```python
from build123d import *

# Parameters (mm, degrees)
F1_DEPTH = 10
F3_DEPTH = 10
F5_D     = 5
F5_DEPTH = 5
F5_TIP   = 1.5021515476


with BuildPart() as f1:
    # F0 (on Top) → F1 (new body)
    with BuildSketch(Plane.XY):
        with BuildLine():
            ThreePointArc((0, 17.5), (12.3743686708, 12.3743686708), (17.5, 0))
            ThreePointArc((17.5, 0), (12.3743686708, -12.3743686708), (0, -17.5))
            Line((0, -17.5), (0, -50))
            Line((0, -50), (150, -50))
            Line((150, -50), (150, 50))
            Line((150, 50), (0, 50))
            Line((0, 50), (0, 17.5))
        make_face()
        with BuildLine():
            ThreePointArc((0, -17.5), (-17.5, 0), (0, 17.5))
            Line((0, 17.5), (0, 50))
            ThreePointArc((0, 50), (-50, 0), (0, -50))
            Line((0, -50), (0, -17.5))
        make_face()
    extrude(amount=F1_DEPTH)

    # F2 (on face) → F3 (join)
    with BuildSketch(Plane.XY.offset(10)):
        with BuildLine():
            Line((150, -25), (150, 25))
            Line((150, 25), (60, 25))
            ThreePointArc((60, 25), (52.9289321881, 22.0710678119), (50, 15))
            Line((50, 15), (50, -15))
            ThreePointArc((50, -15), (52.9289321881, -22.0710678119), (60, -25))
            Line((60, -25), (150, -25))
        make_face()
    extrude(amount=F3_DEPTH)

    # F5
    with Locations(Plane.XY.offset(20)):
        with Locations((60, 15), (70, 15), (80, 15), (60, 5), (70, 5), (80, 5), (60, -5), (70, -5), (80, -5), (60, -15), (70, -15), (80, -15)):
            Hole(F5_D / 2, depth=F5_DEPTH)
            with Locations((0, 0, -(F5_DEPTH + F5_TIP / 2))):  # 118° drill point
                Cone(0, F5_D / 2, F5_TIP, mode=Mode.SUBTRACT)


solid = f1.part
```
Geometry check sheet. Reference: the model listing, model coordinates, mm. A direction names the side the tool comes from. Round coordinates to 2 decimals unless told otherwise and drop trailing zeros. Loops run counter-clockwise (first coordinate to the right, second up) from the corner with the lowest first, then second, coordinate; pieces in that order, holes last. Notation, with made-up numbers: (57, -14) -> (114, -14) arc R17 ccw to (114, 2) -> close; hole circle Ø9 at (39.25, -27.5). An arc over 180 degrees is marked (long way). Use a Markdown table: item, result.
(1) Sectioned sample at B-B (x = -14). Enter the section's corners in (y, z), then the cut area to 3 significant figures.
Calculated:
| item | result |
|---|---|
| outline | (-48, 0) -> (-10.5, 0) -> (-10.5, 10) -> (-48, 10) -> close; (10.5, 0) -> (48, 0) -> (48, 10) -> (10.5, 10) -> close |
| area | 750 mm² |
(2) Scan lines: probe 1 along X at (y, z) = (-15, 17.9); probe 2 along Y at (x, z) = (80, 16.45); probe 3 along Y at (x, z) = (-1, 5). Record each from-to range of solid material in increasing order.
Calculated:
| item | result |
|---|---|
| probe 1 | 50 to 57.5, 62.5 to 67.5, 72.5 to 77.5, 82.5 to 150 |
| probe 2 | -25 to -17.5, -12.5 to -7.5, -2.5 to 2.5, 7.5 to 12.5, 17.5 to 25 |
| probe 3 | -49.99 to -17.47, 17.47 to 49.99 |
(3) Sectioned sample at A-A (z = 17.75). Give the number of separate pieces and of enclosed holes in the cut face, then the cut area to 3 significant figures.
Calculated:
| item | result |
|---|---|
| separate pieces | 1 |
| enclosed holes | 12 |
| area | 4,720 mm² |
(4) Sectioned sample at D-D (x = 103). Enter the section's corners in (y, z), then the cut area to 3 significant figures.
Calculated:
| item | result |
|---|---|
| outline | (-50, 0) -> (50, 0) -> (50, 10) -> (25, 10) -> (25, 20) -> (-25, 20) -> (-25, 10) -> (-50, 10) -> close |
| area | 1,500 mm² |
(5) Set-up check for faces 4 (the flat face through (50, 0, 15)), 5 (the cylindrical face through (53.01, 22.15, 14.93)), 6 (the cylindrical face through (82.5, 5.1, 17.5)), 7 (the flat face through (104, -25, 15)), 8 (the flat face through (76, 50, 5)): record each of +Z, -Z, +X, -X, +Y, -Y from which the full face is reachable in a straight line by a thin tool's end or side.
Calculated:
| item | result |
|---|---|
| face 4 | +Z, -X, +Y, -Y |
| face 5 | +Z, -X, +Y |
| face 6 | +Z |
| face 7 | +Z, +X, -X, -Y |
| face 8 | +Z, -Z, +X, -X, +Y |
(6) Go/stop test with flat-tipped pins: P1, Ø1.5, axis at y = -31, z = 12, coming from the -X side; P2, Ø3, axis at y = 0, z = 14.5, coming from the -X side; P3, Ø4.5, axis at x = 80, y = 15, coming from the +Z side; P4, Ø4, axis at x = 60, y = -15, coming from the +Z side. Record where each tip stops, or that it passes through.
Calculated:
| item | result |
|---|---|
| P1 | through |
| P2 | x = 50 |
| P3 | z = 14.85 |
| P4 | z = 14.7 |
(7) Sectioned sample at C-C (z = 4.5). Enter the section's corners in (x, y).
Calculated:
| item | result |
|---|---|
| outline | (0, -50) -> (150, -50) -> (150, 50) -> (0, 50) arc R50 ccw to start; hole circle Ø35 at (0, 0) |
(8) Mould release check, pull along Y, two halves, no side actions. Record for faces 1 (the cylindrical face through (-49.988, 1.099, 4.93)), 2 (the cylindrical face through (82.5, -4.9, 17.5)), 3 (the cylindrical face through (52.85, -21.99, 14.93)): released by +Y, released by -Y, zero draft, split by the parting line, or undercut.
Calculated:
| item | result |
|---|---|
| face 1 | split by the parting line |
| face 2 | undercut |
| face 3 | released by -Y |
